Could you check a few things on this model? Use its own coordinates, in mm. A direction names the side the tool comes from. Give positions to 0.01 mm unless a question says otherwise; leave off trailing zeros. Loops run counter-clockwise (first coordinate to the right, second up) from the corner with the lowest first, then second, coordinate; pieces in that order, holes last. Notation, with made-up numbers: M -31.75,-23 L 0.25,-23 A21 ccw 0.25,-14 Z; hole C 76,-9 d2. An arc over 180 degrees is marked long. Answer in a Markdown table with one row per item. Add a question column.
```python
from build123d import *

# Parameters (mm, degrees)
MAIN_BRACKET_EXTRUDE_DEPTH        = 54.25
TOP_SCREWHOLE_EXTENSION_DEPTH     = 3
BOTTOM_SCREWHOLE_EXTENSION_DEPTH  = 3
SCREWHOLE_EXTENSION_FILLETS_5MM_R = 5
SKETCH4_R                         = 1.5
TOP_SCREWHOLES_DEPTH              = 8
BOTTOM_START                      = -8
SKETCH5_R                         = 1.5
BOTTOM_SCREWHOLES_DEPTH           = 8
WEIGHT_REDUCTION_DEPTH            = 88.819886832
WEIGHT_REDUCTION_DEPTH_BACK       = 88.819886832


with BuildPart() as part:
    # Sketch1 → Main bracket extrude (new body)
    with BuildSketch(Plane(origin=(0, -6.84807753, 0), x_dir=(1, 0, 0), z_dir=(0, 1, 0))):
        Polygon((-57.75, -74.492924432), (57.75, -94.858690704), (57.75, -91.812410869), (-57.75, -71.446644597), align=None)
    extrude(amount=MAIN_BRACKET_EXTRUDE_DEPTH)

    # Sketch2 → Top screwhole extension (add)
    with BuildSketch(Plane(origin=(0, 47.40192247, 0), x_dir=(1, 0, 0), z_dir=(0, 1, 0))):
        Polygon((-57.75, -74.492924432), (-57.75, -66.369511537), (57.75, -86.735277809), (57.75, -94.858690704), align=None)
    extrude(amount=-TOP_SCREWHOLE_EXTENSION_DEPTH)

    # Sketch3 → Bottom screwhole extension (add)
    with BuildSketch(Plane.XZ.offset(6.84807753)):
        Polygon((-57.75, 74.492924432), (-57.75, 66.369511537), (57.75, 86.735277809), (57.75, 94.858690704), align=None)
    extrude(amount=-BOTTOM_SCREWHOLE_EXTENSION_DEPTH)

    # Screwhole extension fillets 5mm
    screwhole_extension_fillets_5mm_edges = [part.edges().sort_by_distance(p)[0] for p in [
        (0, 44.40192247, 81.629527733),
        (0, -3.84807753, 81.629527733),
    ]]
    fillet(screwhole_extension_fillets_5mm_edges, radius=SCREWHOLE_EXTENSION_FILLETS_5MM_R - 0.0001)  # a hair under: the kernel refuses the full size

    # Sketch4 → Top screwholes (cut)
    with BuildSketch(Plane(origin=(0, 47.40192247, 0), x_dir=(1, 0, 0), z_dir=(0, 1, 0))):
        with Locations(Location((-52.75, -71.312852888, 0), (0, 0, 270))):
            Circle(SKETCH4_R)
        with Locations(Location((0, -80.614101121, 0), (0, 0, 270))):
            Circle(SKETCH4_R)
        with Locations(Location((52.75, -89.915349353, 0), (0, 0, 270))):
            Circle(SKETCH4_R)
    extrude(amount=-TOP_SCREWHOLES_DEPTH, mode=Mode.SUBTRACT)

    # Sketch5 → Bottom screwholes (cut)
    with BuildSketch(Plane.XZ.offset(6.84807753).offset(BOTTOM_START)):
        with Locations(Location((52.75, 89.915349353, 0), (0, 0, 90))):
            Circle(SKETCH5_R)
        with Locations(Location((0, 80.614101121, 0), (0, 0, 90))):
            Circle(SKETCH5_R)
        with Locations(Location((-52.75, 71.312852888, 0), (0, 0, 90))):
            Circle(SKETCH5_R)
    extrude(amount=BOTTOM_SCREWHOLES_DEPTH, mode=Mode.SUBTRACT)

    # Sketch6 → Weight reduction (cut, two sides: drawn at the far end of the back side and taken through both)
    with BuildSketch(Plane(origin=(-14.48041592, 0, 82.12251955), x_dir=(0.9848077530122094, 0, 0.17364817766692336), z_dir=(-0.17364817766692334, 0, 0.9848077530122092)).offset(-WEIGHT_REDUCTION_DEPTH_BACK)):
        with BuildLine():
            Line((-30.93708716, 39.40192247), (4.703799677, 39.40192247))
            ThreePointArc((4.703799677, 39.40192247), (8.239333583, 37.937456376), (9.703799677, 34.40192247))
            Line((9.703799677, 34.40192247), (9.703799677, 6.15192247))
            ThreePointArc((9.703799677, 6.15192247), (8.239333583, 2.616388564), (4.703799677, 1.15192247))
            Line((4.703799677, 1.15192247), (-30.93708716, 1.15192247))
            ThreePointArc((-30.93708716, 1.15192247), (-34.472621066, 2.616388564), (-35.93708716, 6.15192247))
            Line((-35.93708716, 6.15192247), (-35.93708716, 34.40192247))
            ThreePointArc((-35.93708716, 34.40192247), (-34.472621066, 37.937456376), (-30.93708716, 39.40192247))
        make_face()
        with BuildLine():
            Line((24.703799677, 39.40192247), (60.344686513, 39.40192247))
            ThreePointArc((60.344686513, 39.40192247), (63.880220419, 37.937456376), (65.344686513, 34.40192247))
            Line((65.344686513, 34.40192247), (65.344686513, 6.15192247))
            ThreePointArc((65.344686513, 6.15192247), (63.880220419, 2.616388564), (60.344686513, 1.15192247))
            Line((60.344686513, 1.15192247), (24.703799677, 1.15192247))
            ThreePointArc((24.703799677, 1.15192247), (21.168265771, 2.616388564), (19.703799677, 6.15192247))
            Line((19.703799677, 6.15192247), (19.703799677, 34.40192247))
            ThreePointArc((19.703799677, 34.40192247), (21.168265771, 37.937456376), (24.703799677, 39.40192247))
        make_face()
    extrude(amount=WEIGHT_REDUCTION_DEPTH + WEIGHT_REDUCTION_DEPTH_BACK, mode=Mode.SUBTRACT)


solid = part.part
```
Item 1: For faces 4 (the face through (52.175, 44.347, 91.301)), 5 (the face through (-6.141, 37.976, 82.049)), 6 (the face through (0.269, 18.771, 81.677)), 7 (the face through (5.188, 20.079, 84.046)), which set-ups out of +Z, -Z, +X, -X, +Y, -Y let a thin tool reach every point of the face, with its end or its side?
Item 2: I need wall thicknesses on L1, parallel to Y at x = -19, z = 80; L2, parallel to Y at x = 7.5, z = 78.25; L3, parallel to Z at x = 52, y = -4. Which ranges of each line are inside material? Lowest first, please.
Item 3: For P1, Ø2.5, axis at x = -52.75, z = 71.31, coming from the +Y side; P2, Ø8, axis at y = 22, z = 75.5, coming from the +X side, each with a flat end and sliding along its axis, tell me the tip position at first contact or that it passes through.
Item 4: Suppose I cut it at B-B (y = 4). List the corners of the cut face in (x, z) for me, then the cut area to 3 significant figures.
Item 5: If we mould it in two halves opening along X, with no side actions, what happens to faces 1 (the face through (-4.66, 20.47, 82.31)), 2 (the face through (-53.201, -3.681, 72.744)), 3 (the face through (0.873, -3.356, 78.903))? For each: +X half, -X half, draft (parallel to the pull), parting line (faces both ways), or undercut.
Item 6: Suppose I cut it at A-A (y = 22). List the corners of the cut face in (x, z) for me.
Values found:
| question | item | result |
|---|---|---|
| 1 | face 4 | +Y |
| 1 | face 5 | -Z, -X |
| 1 | face 6 | -Z, +X |
| 1 | face 7 | +Z, +X |
| 2 | L1 | -6.85 to 1.15, 39.4 to 47.4 |
| 2 | L2 | -6.85 to -3.83, 44.39 to 47.4 |
| 2 | L3 | 85.72 to 88.62, 91.21 to 93.84 |
| 3 | P1 | y = 39.4 |
| 3 | P2 | x = -49.35 |
| 4 | outline | M -57.75,71.45 L -48.87,73.01 L -49.39,75.97 L -57.75,74.49 Z; M -5.4,83.72 L -4.88,80.77 L 5.92,82.67 L 5.4,85.63 Z; M 49.39,93.38 L 49.91,90.43 L 57.75,91.81 L 57.75,94.86 Z |
| 4 | area | 83.8 mm² |
| 5 | face 1 | -X half |
| 5 | face 2 | undercut |
| 5 | face 3 | +X half |
| 6 | outline | M -57.75,71.45 L -49.35,72.93 L -49.87,75.88 L -57.75,74.49 Z; M -4.92,83.81 L -4.4,80.85 L 5.44,82.59 L 4.92,85.54 Z; M 49.87,93.47 L 50.39,90.52 L 57.75,91.81 L 57.75,94.86 Z |
